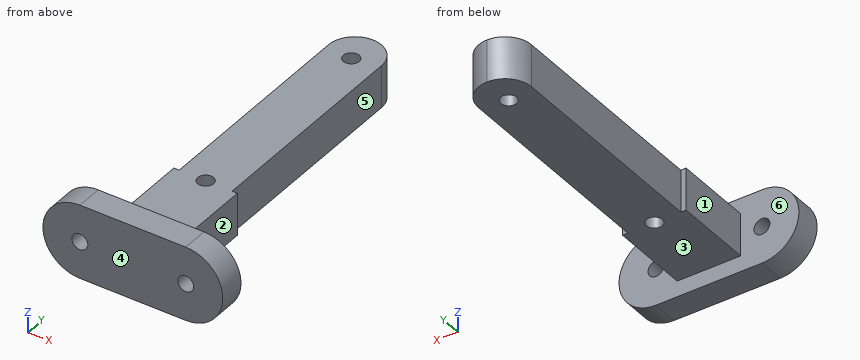
```python
from build123d import *

# Parameters (mm, degrees)
SKETCH1_R           = 1.5
BOSS_EXTRUDE1_DEPTH = 5
SKETCH3_W           = 12
SKETCH3_H           = 8
BOSS_EXTRUDE3_DEPTH = 15
BOSS_EXTRUDE4_START = -8
SKETCH4_W           = 10
SKETCH4_H           = 50.375497142
SKETCH4_R           = 1.5
BOSS_EXTRUDE4_DEPTH = 8
FILLET1_R           = 5
CUT_EXTRUDE1_START  = -8
SKETCH5_R           = 1.5
CUT_EXTRUDE1_DEPTH  = 8


with BuildPart() as part:
    # Sketch1 → Boss-Extrude1 (new body)
    with BuildSketch(Plane(origin=(0, 0, 0), x_dir=(1, 0, 0), z_dir=(0, 1, 0))):
        with BuildLine():
            Line((-10, 6.982882733), (10, 6.982882733))
            ThreePointArc((10, 6.982882733), (16.982882733, 0), (10, -6.982882733))
            Line((10, -6.982882733), (-10, -6.982882733))
            ThreePointArc((-10, -6.982882733), (-16.982882733, 0), (-10, 6.982882733))
        make_face()
        with Locations(Location((-10, 0, 0), (0, 0, 270))):
            Circle(SKETCH1_R, mode=Mode.SUBTRACT)
        with Locations(Location((10, 0, 0), (0, 0, 270))):
            Circle(SKETCH1_R, mode=Mode.SUBTRACT)
    extrude(amount=BOSS_EXTRUDE1_DEPTH)

    # Sketch3 → Boss-Extrude3 (add)
    with BuildSketch(Plane(origin=(0, 5, 0), x_dir=(1, 0, 0), z_dir=(0, 1, 0))):
        Rectangle(SKETCH3_W, SKETCH3_H)
    extrude(amount=BOSS_EXTRUDE3_DEPTH)

    # Sketch4 → Boss-Extrude4 (add)
    with BuildSketch(Plane.XY.offset(4).offset(BOSS_EXTRUDE4_START)):
        with Locations((0, 40.812251429)):
            Rectangle(SKETCH4_W, SKETCH4_H)
        with Locations((0, 20)):
            Circle(SKETCH4_R, mode=Mode.SUBTRACT)
        with Locations((0, 60)):
            Circle(SKETCH4_R, mode=Mode.SUBTRACT)
    extrude(amount=BOSS_EXTRUDE4_DEPTH)

    # Fillet1
    fillet1_edges = [part.edges().sort_by_distance(p)[0] for p in [
        (-5, 66, 0),
        (5, 66, 0),
    ]]
    fillet(fillet1_edges, radius=FILLET1_R - 0.0001)  # a hair under: the kernel refuses the full size

    # Sketch5 → Cut-Extrude1 (cut)
    with BuildSketch(Plane.XY.offset(4).offset(CUT_EXTRUDE1_START)):
        with Locations((0, 20)):
            Circle(SKETCH5_R)
    extrude(amount=CUT_EXTRUDE1_DEPTH, mode=Mode.SUBTRACT)


solid = part.part
```
Verification items for the finished model (mm, model axes). Face numbers are marked on the shaded views. A direction names the side the tool comes from. Coordinates: 2 decimals unless noted, no trailing zeros. Loops run counter-clockwise (first coordinate to the right, second up) from the corner with the lowest first, then second, coordinate; pieces in that order, holes last. Notation, with made-up numbers: (48, 64) - (59, 64) arc R6 ccw to (59, 72) - close; hole circle Ø8 at (-37, 8). An arc over 180 degrees is marked (long way). Answer as a JSON object with one key per item and string values.
(1) Mould release check, pull along Y, two halves, no side actions. Record for the marked faces 4, 5 and 6: pulls with the +Y half, pulls with the -Y half, needs draft (parallel to the pull), parting line crosses it, or undercut.
Response:
{"face 4": "pulls with the -Y half", "face 5": "needs draft", "face 6": "pulls with the +Y half"}
(2) Cross-section at C-C, the plane y = 17. Record the boundary of the cut face in (x, z), then the cut area to 3 significant figures.
Response:
{"outline": "(-6, -4) - (6, -4) - (6, 4) - (-6, 4) - close", "area": "96.0 mm²"}
(3) Cross-section at A-A, the plane z = 0. Count the separate pieces of the cut face and the enclosed holes in it, then the cut area to 3 significant figures.
Response:
{"separate pieces": "3", "enclosed holes": "2", "area": "755 mm²"}
(4) Go/stop test with flat-tipped pins: pin 1 Ø6 at (y, z) = (58.5, 2.5) entering from +X; pin 2 Ø6 at (y, z) = (6.5, -4) entering from +X; pin 3 Ø3.5 at (x, z) = (10, 0) entering from +Y. Record where each tip stops, or that it passes through.
Response:
{"pin 1": "stops at x = 5", "pin 2": "stops at x = 16.84", "pin 3": "stops at y = 5"}
(5) Access from +Z, -Z, +X, -X, +Y, -Y to the whole of each face (thin tool, end or side, straight path). Record for the marked faces 1, 2 and 3.
Response:
{"face 1": "+Z, -Z, -X, +Y", "face 2": "+Z, -Z, +X, +Y", "face 3": "-Z, +X, -X, +Y"}
(6) Cross-section at B-B, the plane y = 60. Record the boundary of the cut face in (x, z).
Response:
{"outline": "(-5, -4) - (-1.5, -4) - (-1.5, 4) - (-5, 4) - close; (1.5, -4) - (5, -4) - (5, 4) - (1.5, 4) - close"}
(7) Cross-section at D-D, the plane x = -7.5. Record the boundary of the cut face in (y, z).
Response:
{"outline": "(0, -6.98) - (5, -6.98) - (5, 6.98) - (0, 6.98) - close"}
(8) Scan lines: line 1 along Y through (x, z) = (0, 0.5); line 2 along X through (y, z) = (3.15, 0); line 3 along Z through (x, y) = (-3, 33). Record each from-to range of solid material in increasing order.
Response:
{"line 1": "y = 0 to 18.5, 21.5 to 58.5, 61.5 to 66", "line 2": "x = -16.98 to -11.5, -8.5 to 8.5, 11.5 to 16.98", "line 3": "z = -4 to 4"}
